CAD build for the part. Positions are in the model's coordinates, mm. Coordinates: 2 decimals unless noted, no trailing zeros. Order: outer loops, then holes, each group sorted by start corner. A loop starts at its lowest first (then second) coordinate and runs counter-clockwise, first axis right, second up.
Autodesk Inventor part; units mm, degrees
ref_plane "YZ Plane" through (0, 0, 0) normal (1, 0, 0) x (0, 1, 0)
ref_plane "XZ Plane" through (0, 0, 0) normal (0, 1, 0) x (-1, 0, 0)
ref_plane "XY Plane" through (0, 0, 0) normal (0, 0, 1) x (1, 0, 0)
sketch "スケッチ1" plane through (0, 0, 0) normal (0, 1, 0) x (-1, 0, 0)
  circle A0 centre (0, 0) radius 5
  dimension "d0" = 10
extrude "押し出し1" add sketch "スケッチ1" along normal blind 2
ref_plane "作業平面1" through (-5.2036, 2.166, -0.9656) normal (0.9686, 0, -0.2487) x (0, -1, 0)
sketch "スケッチ2" plane through (-5.2036, 2.166, -0.9656) normal (0.9686, 0, -0.2487) x (0, -1, 0)
  line L0 (0.166, 2.7706) -> (0.166, -7.2294)
  line L1 (2.166, 2.7706) -> (2.166, -7.2294)
  line L2 (2.166, -7.2294) -> (0.166, -7.2294)
  line L3 (2.166, 2.7706) -> (0.166, 2.7706)
  circle A0 centre (1.166, -1.2294) radius 0.25
  circle A1 centre (1.166, -3.2294) radius 0.25
  point P0 (2.166, -2.2294)
  dimension "d3" = 2
  dimension "d4" = 1
  dimension "d5" = 4
  dimension "d6" = 1
  dimension "d7" = 0.5
  dimension "d8" = 0.5
extrude "押し出し2" cut sketch "スケッチ2" against normal blind 2 contours A0 | A1
properties part number "mini vibrator"
1) Slice it at A-A (x = -3). List the corners of the cut face in (y, z), plus the area to 3 significant figures.
2) Slice it at B-B (y = 0.6). List the corners of the cut face in (x, z).
3) Drill centre lines: probe 1 along Z at (x, y) = (4.25, 0.6); probe 2 along X at (y, z) = (1.25, -1.75); probe 3 along Z at (x, y) = (3.25, 1.5). Where is each one in solid material? Low to high.
4) Slice it at C-C (z = -2.5). List the corners of the cut face in (x, y), plus the area to 3 significant figures.
Worked out:
1. outline: (0, -4) - (2, -4) - (2, 4) - (0, 4) - close
1. area: 16.0 mm2
2. outline: circle Ø10 at (0, 0)
3. probe 1: z = -2.63 to 2.63
3. probe 2: x = -4.68 to 4.68
3. probe 3: z = -3.8 to 3.8
4. outline: (-4.33, 0) - (4.33, 0) - (4.33, 2) - (-4.33, 2) - close
4. area: 17.3 mm2
